from build123d import *

# Parameters (mm, degrees)
SKETCH1_W           = 110
SKETCH1_H           = 15
SKETCH1_W_2         = 70
SKETCH1_H_2         = 5
BOSS_EXTRUDE1_DEPTH = 3
SKETCH2_R           = 1.5
SKETCH2_W           = 3.323826254
SKETCH2_H           = 5
CUT_EXTRUDE1_DEPTH  = 56.590017089


with BuildPart() as part:
    # Sketch1 → Boss-Extrude1 (new body)
    with BuildSketch(Plane(origin=(0, 0, 0), x_dir=(0, 0, -1), z_dir=(1, 0, 0))):
        Rectangle(SKETCH1_W, SKETCH1_H)
        with Locations((0, -0.10154628)):
            Rectangle(SKETCH1_W_2, SKETCH1_H_2, mode=Mode.SUBTRACT)
    extrude(amount=BOSS_EXTRUDE1_DEPTH)

    # Sketch2 → Cut-Extrude1 (cut, through all)
    with BuildSketch(Plane(origin=(3, 0, 0), x_dir=(0, 0, -1), z_dir=(1, 0, 0))):
        with Locations((-45, 0)):
            Circle(SKETCH2_R)
        with Locations((53.338086873, -0.10154628)):
            Rectangle(SKETCH2_W, SKETCH2_H)
    extrude(amount=-CUT_EXTRUDE1_DEPTH, mode=Mode.SUBTRACT)


solid = part.part
The listing builds one solid part. Answer for the finished solid, in the listing's coordinates (mm). A direction names the side the tool comes from. Round coordinates to 2 decimals unless told otherwise and drop trailing zeros. Write each loop counter-clockwise with the first axis right and the second up, starting at its lowest first coordinate (ties: lowest second). Pieces come first, ordered by that corner, then holes. Notation, with made-up numbers: M 71.25,-29.75 L 119.25,-29.75 A13 ccw 119.25,-10.75 Z; hole C 62,27 d11. An arc over 180 degrees is marked long. Write each question's results on one line, items separated by ' | '. Start each with the question number.
Item 1: For faces 1 (the face through (1, 0, 55)), 2 (the face through (2, 0, -51.676)), 3 (the face through (1, 0, 35)), determine the directions among +Z, -Z, +X, -X, +Y, -Y from which every point of the face is accessible in a straight line to the end or side of a thin tool.
Item 2: A cutting plane is placed at C-C on x = 2.1. Write down the section's boundary in (y, z).
Item 3: A cutting plane is placed at D-D on z = 32. Write down the section's boundary in (x, y), and give its area (3 significant figures).
Item 4: A cutting plane is placed at A-A on z = 45. Write down the section's boundary in (x, y).
Item 5: Straight lines are drawn through the part: L1, parallel to Y at x = 0.65, z = 45; L2, parallel to Y at x = 1, z = -14; L3, parallel to Z at x = 0.5, y = -0.75. For each, find the intervals that lie inside material, in ascending order. Write a range as [from, to].
Item 6: A cutting plane is placed at B-B on y = 0. Write down the section's boundary in (x, z), and give its area (3 significant figures).
Item 7: For a pull along Y with two mould halves and no side action, classify faces 4 (the face through (1, -2.602, 0)), 5 (the face through (1, 7.5, 1)), 6 (the face through (3, 3, 1)) as pulls with the +Y half, pulls with the -Y half, needs draft (parallel to the pull), parting line crosses it, or undercut.
Item 8: A flat-ended cylindrical pin translates along its axis: pin 1 Ø1 at (y, z) = (0, -9.5) entering from -X. Find the tip coordinate at first contact, or state that the pin passes through.
Check sheet entries:
1) face 1: +Z, +X, -X, +Y, -Y | face 2: -Z, +X, -X | face 3: +X, -X
2) outline: M -7.5,-55 L -2.6,-55 L -2.6,-51.68 L 2.4,-51.68 L 2.4,-55 L 7.5,-55 L 7.5,55 L -7.5,55 Z; hole M -2.6,-35 L 2.4,-35 L 2.4,35 L -2.6,35 Z; hole C 0,45 d3
3) outline: M 0,-7.5 L 3,-7.5 L 3,-2.6 L 0,-2.6 Z; M 0,2.4 L 3,2.4 L 3,7.5 L 0,7.5 Z | area: 30.0 mm²
4) outline: M 0,-7.5 L 3,-7.5 L 3,-1.5 L 0,-1.5 Z; M 0,1.5 L 3,1.5 L 3,7.5 L 0,7.5 Z
5) L1: [-7.5, -1.5], [1.5, 7.5] | L2: [-7.5, -2.6], [2.4, 7.5] | L3: [-51.68, -35], [35, 43.7], [46.3, 55]
6) outline: M 0,-51.68 L 3,-51.68 L 3,-35 L 0,-35 Z; M 0,35 L 3,35 L 3,43.5 L 0,43.5 Z; M 0,46.5 L 3,46.5 L 3,55 L 0,55 Z | area: 101 mm²
7) face 4: undercut | face 5: pulls with the +Y half | face 6: needs draft
8) pin 1: through
